Could you check a few things on this model? Use its own coordinates, in mm. Face numbers are marked on the shaded views. A direction names the side the tool comes from. Round coordinates to 2 decimals unless told otherwise and drop trailing zeros. Loops run counter-clockwise (first coordinate to the right, second up) from the corner with the lowest first, then second, coordinate; pieces in that order, holes last. Notation, with made-up numbers: (-36, 67) - (-7, 67) arc R30 cw to (-7, 103) - close; hole circle Ø7 at (61, 64.5). An arc over 180 degrees is marked (long way). Use one line per item in the form item = value.
```python
from build123d import *

# Parameters (mm, degrees)
F0_W     = 7.7755046077
F0_H     = 1.5709503787
F1_DEPTH = 8
F2_W     = 7.7755046077
F2_H     = 6.0012028553
F3_DEPTH = 8
F4_R     = 2.8924366319
F4_R_2   = 2.4816180031
F5_DEPTH = 1.9
F6_R     = 2.2667202486
F7_DEPTH = 1.5


with BuildPart() as f1:
    # F0 (on Front) → F1 (new body)
    with BuildSketch(Plane.XZ):
        with Locations((3.8877523039, 0.7854751893)):
            Rectangle(F0_W, F0_H)
    extrude(amount=F1_DEPTH)

    # F2 (on face) → F3 (join)
    with BuildSketch(Plane.XY.offset(1.5709503787)):
        with Locations((3.8877523039, -3.0006014276)):
            Rectangle(F2_W, F2_H)
    extrude(amount=F3_DEPTH)

    # F4 (on face) → F5 (join)
    with BuildSketch(Plane.XZ.offset(6.0012028553)):
        with Locations((3.8877523039, 5.5709503787)):
            Circle(F4_R)
        with Locations((3.8877523039, 5.5709503787)):
            Circle(F4_R_2, mode=Mode.SUBTRACT)
    extrude(amount=F5_DEPTH)

    # F6 (on face) → F7 (join)
    with BuildSketch(Plane.XY.offset(9.5709503787)):
        with Locations((3.8877523039, -3.0006014276)):
            Circle(F6_R)
    extrude(amount=F7_DEPTH)


solid = f1.part
```
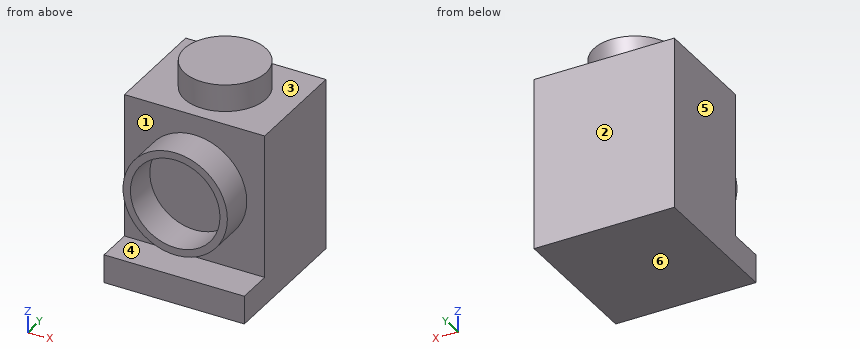
1. If we section it at B-B, the plane x = 2.5: Write out the boundary of the cut face in (y, z), plus the area to 3 significant figures.
Solution:
outline = (-8, 0) - (0, 0) - (0, 9.57) - (-1.21, 9.57) - (-1.21, 11.07) - (-4.79, 11.07) - (-4.79, 9.57) - (-6, 9.57) - (-6, 8.11) - (-7.9, 8.11) - (-7.9, 7.63) - (-6, 7.63) - (-6, 3.51) - (-7.9, 3.51) - (-7.9, 3.03) - (-6, 3.03) - (-6, 1.57) - (-8, 1.57) - close
area = 67.8 mm^2
2. Please list where these lines run through material, in increasing order: line 1 along Z through (x, y) = (4.25, -7.25); line 2 along Z through (x, y) = (3, -6.5); line 3 along Z through (x, y) = (1, -2).
Solution:
line_1 = 0 to 1.57, 2.7 to 3.12, 8.03 to 8.44
line_2 = 0 to 1.57, 2.82 to 3.25, 7.89 to 8.32
line_3 = 0 to 9.57
3. If we section it at A-A, the plane y = -6.75: Write out the boundary of the cut face in (x, z), plus the area to 3 significant figures.
Solution:
outline = (0, 0) - (7.78, 0) - (7.78, 1.57) - (0, 1.57) - close; circle Ø5.78 at (3.89, 5.57); hole circle Ø4.96 at (3.89, 5.57)
area = 19.2 mm^2
4. If we section it at C-C, the plane y = -2.25: Write out the boundary of the cut face in (x, z).
Solution:
outline = (0, 0) - (7.78, 0) - (7.78, 9.57) - (6.03, 9.57) - (6.03, 11.07) - (1.75, 11.07) - (1.75, 9.57) - (0, 9.57) - close
5. On a 3-axis mill with a long thin cutter (end or side, diameter ignored), from which of +Z, -Z, +X, -X, +Y, -Y can I reach the whole of each face in a straight line? I mean the marked faces 1, 2 and 3. Say none if no direction works.
Solution:
face_1 = -Y
face_2 = +Z, -Z, +X, -X, +Y
face_3 = +Z
6. We'd pull the mould along Z, two halves only. Please class the marked faces 4, 5 and 6: +Z half, -Z half, draft (parallel to the pull), parting line (faces both ways), or undercut.
Solution:
face_4 = undercut
face_5 = draft
face_6 = -Z half
7. For P1, Ø3, axis at x = 5, z = 5, coming from the -Y side; P2, Ø1.6, axis at x = 5, y = -7, coming from the +Z side, each with a flat end and sliding along its axis, tell me the tip position at first contact or that it passes through.
Solution:
P1 = -7.9
P2 = 8.45
8. If we section it at D-D, the plane z = 5: Write out the boundary of the cut face in (x, y).
Solution:
outline = (0, -6) - (1.05, -6) - (1.05, -7.9) - (1.47, -7.9) - (1.47, -6) - (6.3, -6) - (6.3, -7.9) - (6.72, -7.9) - (6.72, -6) - (7.78, -6) - (7.78, 0) - (0, 0) - close
